```python
from build123d import *

# Parameters (mm, degrees)
SKETCH1_W           = 2.92
SKETCH1_H           = 2.92
SKETCH1_R           = 2.52
SKETCH1_R_2         = 0.5
BOSS_EXTRUDE1_DEPTH = 3


with BuildPart() as part:
    # Sketch1 → Boss-Extrude1 (new body)
    with BuildSketch(Plane.XY):
        Polygon((13.5482559, 6.709731544), (8.5482559, 11.709731544), (-2.4517441, 11.709731544), (-7.4517441, 6.709731544), (-7.4517441, -13.790268456), (13.5482559, -13.790268456), align=None)
        with Locations((3.0482559, -3.330268456)):
            Rectangle(SKETCH1_W, SKETCH1_H, mode=Mode.SUBTRACT)
        with Locations((3.0482559, 2.709731544)):
            Circle(SKETCH1_R, mode=Mode.SUBTRACT)
        with Locations((3.0482559, 8.709731544)):
            Circle(SKETCH1_R_2, mode=Mode.SUBTRACT)
    extrude(amount=BOSS_EXTRUDE1_DEPTH)


solid = part.part
```
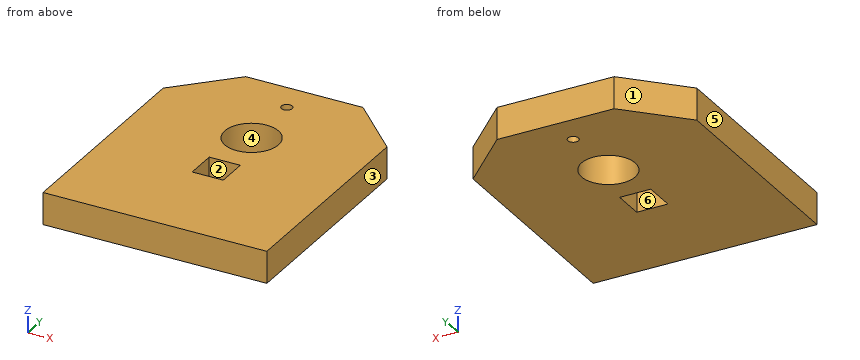
Work out the finished part from the listing and answer in its coordinate system (mm). Face numbers are marked on the shaded views. A direction names the side the tool comes from. Give positions to 0.01 mm unless a question says otherwise; leave off trailing zeros. Order: outer loops, then holes, each group sorted by start corner. A loop starts at its lowest first (then second) coordinate and runs counter-clockwise, first axis right, second up. Notation, with made-up numbers: (82.5, 12) - (92.5, 12) arc R11 cw to (92.5, 33) - close; hole circle Ø8 at (-19, 43.25). An arc over 180 degrees is marked (long way). One line per item, written item: value. Start each with the question number.
1. Section B-B, the plane x = 2.25 is taken. Write down the section's boundary in (y, z).
2. Which of the six approach directions +Z, -Z, +X, -X, +Y, -Y give full straight-line access (tool end or side, diameter ignored) to the marked faces 5 and 6?
3. Consider line 1 (X direction, y = 2.75, z = 2.7); line 2 (X direction, y = -4, z = 2.8); line 3 (Y direction, x = 1.75, z = 1.5). Determine where each line is inside the solid, lowest interval first.
4. This flat-tipped pin is pushed along its axis until it touches: pin 1 Ø1.5 at (x, z) = (-4, 1) entering from +Y. Where does it stop, or does it pass through?
5. For a pull along Y with two mould halves and no side action, classify the marked faces 1, 2, 3 and 4 as released by +Y, released by -Y, zero draft, split by the parting line, or undercut.
6. Section C-C, the plane z = 0.4 is taken. Write down the section's boundary in (x, y), then the cut area to 3 significant figures.
7. Section D-D, the plane x = -4.75 is taken. Write down the section's boundary in (y, z), then the cut area to 3 significant figures.
8. Section A-A, the plane y = 3.5 is taken. Write down the section's boundary in (x, z), then the cut area to 3 significant figures.
Filled sheet:
1. outline: (-13.79, 0) - (-4.79, 0) - (-4.79, 3) - (-13.79, 3) - close; (-1.87, 0) - (0.32, 0) - (0.32, 3) - (-1.87, 3) - close; (5.1, 0) - (11.71, 0) - (11.71, 3) - (5.1, 3) - close
2. face 5: +Z, -Z, -X, +Y, -Y
2. face 6: +Z, -Z
3. line 1: -7.45 to 0.53, 5.57 to 13.55
3. line 2: -7.45 to 1.59, 4.51 to 13.55
3. line 3: -13.79 to -4.79, -1.87 to 0.55, 4.87 to 11.71
4. pin 1: y = 10.91
5. face 1: released by +Y
5. face 2: undercut
5. face 3: zero draft
5. face 4: undercut
6. outline: (-7.45, -13.79) - (13.55, -13.79) - (13.55, 6.71) - (8.55, 11.71) - (-2.45, 11.71) - (-7.45, 6.71) - close; hole circle Ø5.04 at (3.05, 2.71); hole (1.59, -4.79) - (4.51, -4.79) - (4.51, -1.87) - (1.59, -1.87) - close; hole circle Ø1 at (3.05, 8.71)
6. area: 481 mm²
7. outline: (-13.79, 0) - (9.41, 0) - (9.41, 3) - (-13.79, 3) - close
7. area: 69.6 mm²
8. outline: (-7.45, 0) - (0.66, 0) - (0.66, 3) - (-7.45, 3) - close; (5.44, 0) - (13.55, 0) - (13.55, 3) - (5.44, 3) - close
8. area: 48.6 mm²
